```python
from build123d import *

# Parameters (mm, degrees)
PAD_DEPTH       = 35
POCKET001_DEPTH = 4.501
SKETCH010_R     = 2.1
POCKET_DEPTH    = 4.501


with BuildPart() as part:
    # Sketch001 → Pad (new body)
    with BuildSketch(Plane(origin=(0, 2.56, 3.75), x_dir=(1, 0, 0), z_dir=(0, -1, 0))):
        Polygon((-3.2, 0), (1, 0), (1, 3.3), (-0.5, 5.3), (-0.5, 25), (-4.5, 24.8), (-4.5, 4.7), (-3.2, 4.7), align=None)
    extrude(amount=PAD_DEPTH)

    # Sketch004 (on Body) → Pocket001 (cut, through all)
    with BuildSketch(Plane(origin=(0, 0.1, 0), x_dir=(0, 1, 0), z_dir=(1, 0, 0))):
        Polygon((-0.374562, 28.780826), (2.525438, 25.880826), (2.525438, 28.780826), align=None)
    extrude(amount=-POCKET001_DEPTH, mode=Mode.SUBTRACT)

    # Sketch010 → Pocket (cut, through all)
    with BuildSketch(Plane.YZ):
        with Locations((-14.943965, 19.475978)):
            Circle(SKETCH010_R)
    extrude(amount=-POCKET_DEPTH, mode=Mode.SUBTRACT)


solid = part.part
```
Source: CAD feature listing. Evaluate the final solid. Frame: model axes, mm. A direction names the side the tool comes from. Give positions to 0.01 mm unless a question says otherwise; leave off trailing zeros. Order: outer loops, then holes, each group sorted by start corner. A loop starts at its lowest first (then second) coordinate and runs counter-clockwise, first axis right, second up.
(1) Pull-direction query (Y, two-part tool) for faces 4 (the face through (-2.5, -14, 17.6)), 5 (the face through (-2, -32.44, 16)), 6 (the face through (-4, -15, 8.45)); classes: +Y half, -Y half, draft (parallel to the pull), parting line (faces both ways), or undercut.
(2) Section query D-D (z = 6.5). Return the cut outline in (x, y), plus the area to 3 significant figures.
(3) Access query for faces 1 (the face through (-3.2, -15, 6)), 2 (the face through (1, -15, 5)), 3 (the face through (-0.5, -15, 17)). Directions: +Z, -Z, +X, -X, +Y, -Y. A direction counts if a zero-diameter tool reaches every point of the face in a straight line with its end or side. Return the directions, or none.
(4) Section query C-C (z = 18.75). Return the cut outline in (x, y), plus the area to 3 significant figures.
(5) Section query B-B (x = -2.75). Return the cut outline in (y, z).
(6) Material intervals for line 1 along X through (y, z) = (-24.5, 15.5); line 2 along Z through (x, y) = (-0.9, -16.5); line 3 along Z through (x, y) = (-0.6, -17.5) (3 decimals), sorted ascending.
(7) Section query A-A (y = -22). Return the cut outline in (x, z).
(8) Contact query for flat-ended pins moving along their axis: P1, Ø6, axis at y = -12.5, z = 23, coming from the +X side; P2, Ø1.5, axis at x = -1.5, y = -24.5, coming from the +Z side; P3, Ø5, axis at y = -14.94, z = 19.48, coming from the -X side. Output: stop coordinate, or through.
Outcome:
1. face 4: undercut
1. face 5: -Y half
1. face 6: draft
2. outline: (-3.2, -32.44) - (1, -32.44) - (1, 2.56) - (-3.2, 2.56) - close
2. area: 147 mm2
3. face 1: -Z, -X, +Y, -Y
3. face 2: +Z, -Z, +X, +Y, -Y
3. face 3: +Z, +X, +Y, -Y
4. outline: (-4.5, -32.44) - (-0.5, -32.44) - (-0.5, -16.91) - (-4.5, -16.91) - close; (-4.5, -12.97) - (-0.5, -12.97) - (-0.5, 2.56) - (-4.5, 2.56) - close
4. area: 124 mm2
5. outline: (-32.44, 3.75) - (2.56, 3.75) - (2.56, 25.95) - (-0.13, 28.64) - (-32.44, 28.64) - close; hole circle Ø4.2 at (-14.94, 19.48)
6. line 1: x = -4.5 to -0.5
6. line 2: z = 3.75 to 18.07, 20.89 to 28.73
6. line 3: z = 3.75 to 28.745
7. outline: (-4.5, 8.45) - (-3.2, 8.45) - (-3.2, 3.75) - (1, 3.75) - (1, 7.05) - (-0.5, 9.05) - (-0.5, 28.75) - (-4.5, 28.55) - close
8. P1: stops at x = -0.5
8. P2: stops at z = 28.74
8. P3: stops at x = -4.5
